Read the model definition and answer for the solid it produces. Units are mm, in the model's axes. A direction names the side the tool comes from. Coordinates: 2 decimals unless noted, no trailing zeros. Write each loop counter-clockwise with the first axis right and the second up, starting at its lowest first coordinate (ties: lowest second). Pieces come first, ordered by that corner, then holes.
(1) Straight lines are drawn through the part: line 1 along Z through (x, y) = (1, -8.5); line 2 along Z through (x, y) = (5.75, 8.25); line 3 along Y through (x, z) = (9.75, 32.5). For each, find the intervals that lie inside material, in ascending order.
(2) The part is cut by section A-A, the plane z = 22.5. Determine the outline of the cut face in (x, y), and give its area (3 significant figures).
(3) Which of the six approach directions +Z, -Z, +X, -X, +Y, -Y give full straight-line access (tool end or side, diameter ignored) to faces 1 (the flat face through (8, -6, 0)), 2 (the cylindrical face through (10.62, 3.34, 32.29)), 3 (the flat face through (-1.9, 5.4, 64.061))?
(4) Given pin 1 (8 mm diameter, centred on x = -5, z = 19.5, fed in from +Y); pin 2 (1 mm diameter, centred on y = -1, z = 42, fed in from -X); pin 3 (1 mm diameter, centred on x = 2, z = 12.5, fed in from +Y); pin 4 (11 mm diameter, centred on x = 5.5, y = 3.5, fed in from +Z), each flat-ended and moving along its own axis, determine where each tip first touches the part or whether it passes through.
```python
from build123d import *

# Parameters (mm, degrees)
F0_W = 5.566528
F0_H = 0.37384


with BuildPart() as f1:
    # F0 (on Front) → F1 (revolve)
    with BuildSketch(Plane.XZ):
        with BuildLine():
            Line((0, 64.957067), (0, 64.06147))
            Line((0, 64.06147), (5.566528, 64.06147))
            Line((5.566528, 64.06147), (5.566528, 64.776555))
            ThreePointArc((5.566528, 64.776555), (5.513657, 64.904197), (5.386015, 64.957067))
            Line((5.386015, 64.957067), (0, 64.957067))
        make_face()
        with Locations((2.783264, 63.87455)):
            Rectangle(F0_W, F0_H)
        with BuildLine():
            Line((5.566528, 64.06147), (5.566528, 63.68763))
            Line((5.566528, 63.68763), (8.045916, 63.68763))
            Line((8.045916, 63.68763), (8.045916, 63.880958))
            ThreePointArc((8.045916, 63.880958), (7.993046, 64.008599), (7.865404, 64.06147))
            Line((7.865404, 64.06147), (5.566528, 64.06147))
        make_face()
        with BuildLine():
            Line((0, 63.68763), (0, 0))
            Line((0, 0), (9.809786, 0))
            Line((9.809786, 0), (10.952543, 0))
            ThreePointArc((10.952543, 0), (11.080184, 0.052871), (11.133055, 0.180512))
            Line((11.133055, 0.180512), (11.133055, 63.507118))
            ThreePointArc((11.133055, 63.507118), (11.080184, 63.634759), (10.952543, 63.68763))
            Line((10.952543, 63.68763), (8.045916, 63.68763))
            Line((8.045916, 63.68763), (5.566528, 63.68763))
            Line((5.566528, 63.68763), (0, 63.68763))
        make_face()
        with BuildLine():
            Line((9.809786, 0), (0, 0))
            Line((0, 0), (0, -0.365171))
            Line((0, -0.365171), (9.629273, -0.365171))
            ThreePointArc((9.629273, -0.365171), (9.756915, -0.3123), (9.809786, -0.184658))
            Line((9.809786, -0.184658), (9.809786, 0))
        make_face()
    revolve(axis=Axis((0, 0, 31.843815), (0, 0, 1)))


solid = f1.part
```
Computed:
1. line 1: z = -0.37 to 63.69
1. line 2: z = 0 to 63.69
1. line 3: y = -5.37 to 5.37
2. outline: circle Ø22.27 at (0, 0)
2. area: 389 mm2
3. face 1: -Z
3. face 2: +Z, -Z
3. face 3: +Z
4. pin 1: stops at y = 11.09
4. pin 2: stops at x = -11.12
4. pin 3: stops at y = 11.03
4. pin 4: stops at z = 64.96
